from build123d import *

# Parameters (mm, degrees)
BOSS_EXTRUDE1_DEPTH     = 150
CUT_EXTRUDE5_DEPTH      = 153.060765161
CUT_EXTRUDE6_DEPTH      = 153.060765161
CUT_EXTRUDE6_DEPTH_BACK = 153.060765161
SKETCH3_R               = 2
CUT_EXTRUDE7_DEPTH      = 153.060765161
CUT_EXTRUDE7_DEPTH_BACK = 153.060765161
SKETCH6_R               = 2


with BuildPart() as part:
    # Sketch1 → Boss-Extrude1 (new body)
    with BuildSketch(Plane.XY):
        with BuildLine():
            Line((4.445, 18.415), (5.6388, 18.415))
            Line((5.6388, 18.415), (5.6388, 21.294464083))
            ThreePointArc((5.6388, 21.294464083), (5.173007463, 22.391174147), (4.060357789, 22.817491346))
            Line((4.060357789, 22.817491346), (0.743323143, 22.698920454))
            Line((0.743323143, 22.698920454), (-3.892452069, 22.8203125))
            ThreePointArc((-3.892452069, 22.8203125), (-5.124499805, 22.338098312), (-5.6388, 21.119095664))
            Line((-5.6388, 21.119095664), (-5.6388, -21.119095664))
            ThreePointArc((-5.6388, -21.119095664), (-5.124499805, -22.338098312), (-3.892452069, -22.8203125))
            Line((-3.892452069, -22.8203125), (0.743323143, -22.698920454))
            Line((0.743323143, -22.698920454), (4.060357789, -22.817491346))
            ThreePointArc((4.060357789, -22.817491346), (5.173007463, -22.391174147), (5.6388, -21.294464083))
            Line((5.6388, -21.294464083), (5.6388, -18.415))
            Line((5.6388, -18.415), (4.445, -18.415))
            Line((4.445, -18.415), (4.445, -21.3734366))
            ThreePointArc((4.445, -21.3734366), (4.367367911, -21.55622161), (4.181926298, -21.627274477))
            Line((4.181926298, -21.627274477), (1.131158407, -21.51822157))
            ThreePointArc((1.131158407, -21.51822157), (0.187154328, -21.71413397), (-0.761857041, -21.544125758))
            Line((-0.761857041, -21.544125758), (-3.92370211, -21.626921585))
            ThreePointArc((-3.92370211, -21.626921585), (-4.291477554, -21.482977052), (-4.445, -21.119095664))
            Line((-4.445, -21.119095664), (-4.445, 21.119095664))
            ThreePointArc((-4.445, 21.119095664), (-4.291477554, 21.482977052), (-3.92370211, 21.626921585))
            Line((-3.92370211, 21.626921585), (-0.761857041, 21.544125758))
            ThreePointArc((-0.761857041, 21.544125758), (0.187154328, 21.71413397), (1.131158407, 21.51822157))
            Line((1.131158407, 21.51822157), (4.191, 21.6274366))
            ThreePointArc((4.191, 21.6274366), (4.370605122, 21.553041722), (4.445, 21.3734366))
            Line((4.445, 21.3734366), (4.445, 18.415))
        make_face()
    extrude(amount=BOSS_EXTRUDE1_DEPTH)

    # Sketch2 → Cut-Extrude5 (cut, through all)
    with BuildSketch(Plane(origin=(-4.445, 0, 0), x_dir=(0, 0, -1), z_dir=(1, 0, 0))):
        with BuildLine():
            Line((-150.086983229, 12.208813289), (-150.086983229, -12.200691478))
            Line((-150.086983229, -12.200691478), (-140.690340072, -12.200691478))
            ThreePointArc((-140.690340072, -12.200691478), (-138.407548952, -10.035772864), (-140.448517226, -7.641517989))
            Line((-140.448517226, -7.641517989), (-141.882783229, -7.4889391))
            Line((-141.882783229, -7.4889391), (-141.882783229, 7.497060911))
            Line((-141.882783229, 7.497060911), (-140.448517226, 7.6496398))
            ThreePointArc((-140.448517226, 7.6496398), (-138.407548952, 10.043894675), (-140.690340072, 12.208813289))
            Line((-140.690340072, 12.208813289), (-150.086983229, 12.208813289))
        make_face()
    extrude(amount=-CUT_EXTRUDE5_DEPTH, mode=Mode.SUBTRACT)

    # Sketch3 → Cut-Extrude6 (cut, two sides: drawn at the far end of the back side and taken through both)
    with BuildSketch(Plane(origin=(-4.445, 0, 0), x_dir=(0, 0, -1), z_dir=(1, 0, 0)).offset(-CUT_EXTRUDE6_DEPTH_BACK)):
        with Locations(Location((-83.046273188, -0.038624064, 0), (0, 0, 90))):
            Circle(SKETCH3_R)
        with BuildLine():
            Line((-105.612723982, 10.28792521), (-79.030103641, 10.28792521))
            ThreePointArc((-79.030103641, 10.28792521), (-77.422829038, 8.680650607), (-79.030103641, 7.073376004))
            Line((-79.030103641, 7.073376004), (-101.174207902, 7.073376004))
            ThreePointArc((-101.174207902, 7.073376004), (-102.251838636, 6.627006739), (-102.698207902, 5.549376004))
            Line((-102.698207902, 5.549376004), (-102.698207902, -5.626624133))
            ThreePointArc((-102.698207902, -5.626624133), (-102.251199404, -6.70579811), (-101.172025428, -7.152806607))
            Line((-101.172025428, -7.152806607), (-79.030103641, -7.152806607))
            ThreePointArc((-79.030103641, -7.152806607), (-77.443694877, -8.73921537), (-79.030103641, -10.325624133))
            Line((-79.030103641, -10.325624133), (-105.652273188, -10.325624133))
            ThreePointArc((-105.652273188, -10.325624133), (-106.729903922, -9.879254868), (-107.176273188, -8.801624133))
            Line((-107.176273188, -8.801624133), (-107.176273188, 8.724376004))
            ThreePointArc((-107.176273188, 8.724376004), (-106.718320228, 9.82997225), (-105.612723982, 10.28792521))
        make_face()
        with BuildLine():
            Line((-96.952773188, 2.247375936), (-91.999773188, 2.247375936))
            ThreePointArc((-91.999773188, 2.247375936), (-89.999773188, 0.247375936), (-91.999773188, -1.752624064))
            Line((-91.999773188, -1.752624064), (-96.952773188, -1.752624064))
            ThreePointArc((-96.952773188, -1.752624064), (-98.952773188, 0.247375936), (-96.952773188, 2.247375936))
        make_face()
    extrude(amount=CUT_EXTRUDE6_DEPTH + CUT_EXTRUDE6_DEPTH_BACK, mode=Mode.SUBTRACT)

    # Sketch6 → Cut-Extrude7 (cut, two sides: drawn at the far end of the back side and taken through both)
    with BuildSketch(Plane(origin=(-4.445, 0, 0), x_dir=(0, 0, -1), z_dir=(1, 0, 0)).offset(-CUT_EXTRUDE7_DEPTH_BACK)):
        with Locations(Location((-40.899819498, -0.049300509, 0), (0, 0, 90))):
            Circle(SKETCH6_R)
        with BuildLine():
            Line((-18.333368704, -10.375849783), (-44.915989045, -10.375849783))
            ThreePointArc((-44.915989045, -10.375849783), (-46.523263648, -8.76857518), (-44.915989045, -7.161300577))
            Line((-44.915989045, -7.161300577), (-22.771884784, -7.161300577))
            ThreePointArc((-22.771884784, -7.161300577), (-21.694254049, -6.714931312), (-21.247884784, -5.637300577))
            Line((-21.247884784, -5.637300577), (-21.247884784, 5.53869956))
            ThreePointArc((-21.247884784, 5.53869956), (-21.694893281, 6.617873536), (-22.774067257, 7.064882034))
            Line((-22.774067257, 7.064882034), (-44.915989045, 7.064882034))
            ThreePointArc((-44.915989045, 7.064882034), (-46.502397808, 8.651290797), (-44.915989045, 10.23769956))
            Line((-44.915989045, 10.23769956), (-18.293819498, 10.23769956))
            ThreePointArc((-18.293819498, 10.23769956), (-17.216188763, 9.791330295), (-16.769819498, 8.71369956))
            Line((-16.769819498, 8.71369956), (-16.769819498, -8.812300577))
            ThreePointArc((-16.769819498, -8.812300577), (-17.227772458, -9.917896824), (-18.333368704, -10.375849783))
        make_face()
        with BuildLine():
            Line((-26.993319498, -1.763300509), (-31.946319498, -1.763300509))
            ThreePointArc((-31.946319498, -1.763300509), (-33.946319498, 0.236699491), (-31.946319498, 2.236699491))
            Line((-31.946319498, 2.236699491), (-26.993319498, 2.236699491))
            ThreePointArc((-26.993319498, 2.236699491), (-24.993319498, 0.236699491), (-26.993319498, -1.763300509))
        make_face()
    extrude(amount=CUT_EXTRUDE7_DEPTH + CUT_EXTRUDE7_DEPTH_BACK, mode=Mode.SUBTRACT)


solid = part.part
Design review of the part built by this model. Coordinates are the model's own, in mm. A direction names the side the tool comes from. Give positions to 0.01 mm unless a question says otherwise; leave off trailing zeros. Write each loop counter-clockwise with the first axis right and the second up, starting at its lowest first coordinate (ties: lowest second). Pieces come first, ordered by that corner, then holes. Notation, with made-up numbers: M 11.25,86 L 45.25,86 A25 ccw 45.25,119 Z; hole C 71,30 d10. An arc over 180 degrees is marked long. Answer as a JSON object with one key per item and string values. Group by question number.
1) For line 1 along Y through (x, z) = (-3.25, 134); line 2 along Y through (x, z) = (1.5, 142); line 3 along X through (y, z) = (-19.5, 40.5) (3 decimals), list the stretches that pass through material, from the lowest coordinate up.
2) We need section C-C (y = 13.5). Give the boundary of the cut face in (x, z) (3 decimals), and give its area (3 significant figures).
3) Mouldability with a two-part tool opening along Z and no side actions: class faces 3 (the face through (-5.05, 0.874, 39.125)), 4 (the face through (-1, -22, 150)), 5 (the face through (-5.639, 0, 74)) as released by +Z, released by -Z, zero draft, split by the parting line, or undercut.
4) Clearance check with flat-ended pins moving along their axes: pin 1 Ø0.6 at (x, z) = (-5, 88) entering from -Y; pin 2 Ø2 at (x, z) = (2.5, 135) entering from -Y; pin 3 Ø2 at (x, z) = (1, 109) entering from -Y. State where each tip first meets the part, or that it passes through.
5) Tool access review of faces 1 (the face through (4.445, 20, 74)), 2 (the face through (-5, -2, 0)): name each direction out of +Z, -Z, +X, -X, +Y, -Y from which nothing blocks a thin tool from reaching the whole face with its end or side.
6) We need section A-A (y = 0.5). Give the boundary of the cut face in (x, z) (3 decimals).
Answer key:
{
 "1": {"line 1": "y = -22.8 to -21.61, 21.61 to 22.8", "line 2": "y = -22.73 to -21.53, 21.53 to 22.73", "line 3": "x = -5.639 to -4.445, 4.445 to 5.639"},
 "2": {"outline": "M -5.639,0 L -4.445,0 L -4.445,150 L -5.639,150 Z", "area": "179 mm²"},
 "3": {"face 3": "undercut", "face 4": "released by +Z", "face 5": "zero draft"},
 "4": {"pin 1": "stops at y = -22.64", "pin 2": "stops at y = -22.8", "pin 3": "stops at y = -22.74"},
 "5": {"face 1": "+Z, -Z", "face 2": "-Z, +X, -X, +Y, -Y"},
 "6": {"outline": "M -5.639,0 L -4.445,0 L -4.445,16.77 L -5.639,16.77 Z; M -5.639,21.248 L -4.445,21.248 L -4.445,25.011 L -5.639,25.011 Z; M -5.639,33.929 L -4.445,33.929 L -4.445,38.977 L -5.639,38.977 Z; M -5.639,42.823 L -4.445,42.823 L -4.445,81.12 L -5.639,81.12 Z; M -5.639,84.972 L -4.445,84.972 L -4.445,90.016 L -5.639,90.016 Z; M -5.639,98.937 L -4.445,98.937 L -4.445,102.698 L -5.639,102.698 Z; M -5.639,107.176 L -4.445,107.176 L -4.445,141.883 L -5.639,141.883 Z"}
}
